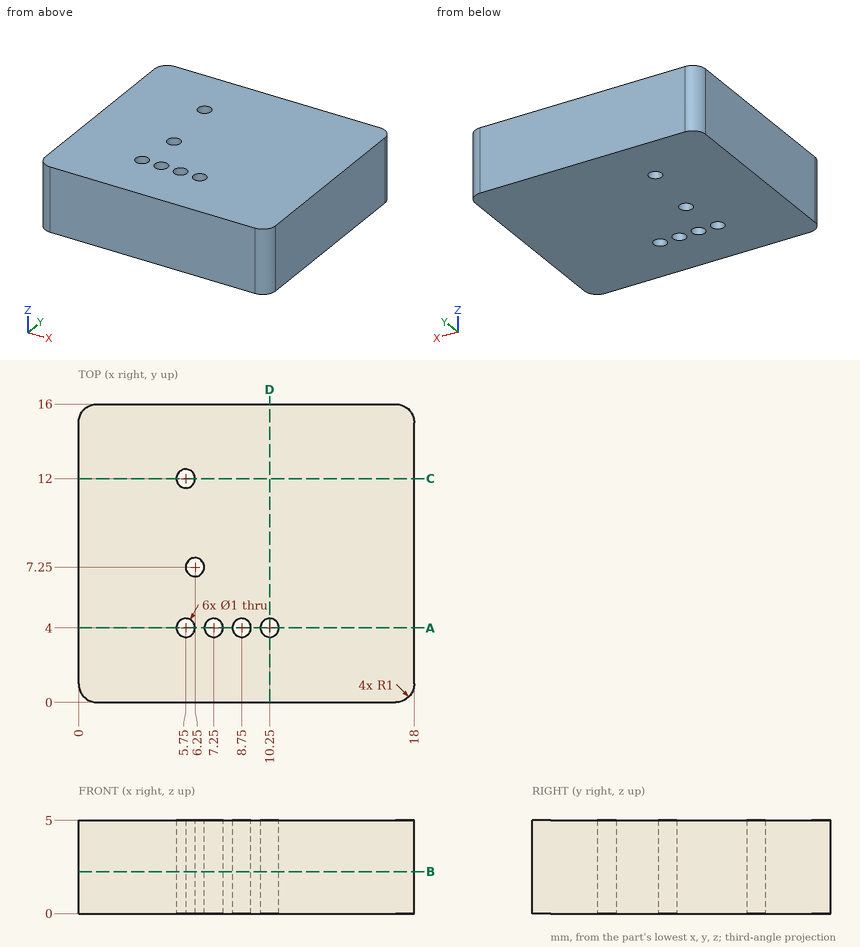
Job drawing, mm, ordinate dimensions from the low corner. One solid piece. Give positions to 0.01 mm unless a question says otherwise; leave off trailing zeros. Loops run counter-clockwise (first coordinate to the right, second up) from the corner with the lowest first, then second, coordinate; pieces in that order, holes last.
Item 1: Slice it at A-A, the plane y = 4. List the corners of the cut face in (x, z).
Answers follow:
outline: (0, 0) - (5.25, 0) - (5.25, 5) - (0, 5) - close; (6.25, 0) - (6.75, 0) - (6.75, 5) - (6.25, 5) - close; (7.75, 0) - (8.25, 0) - (8.25, 5) - (7.75, 5) - close; (9.25, 0) - (9.75, 0) - (9.75, 5) - (9.25, 5) - close; (10.75, 0) - (18, 0) - (18, 5) - (10.75, 5) - close
Item 2: Slice it at D-D, the plane x = 10.25. List the corners of the cut face in (y, z), and give its area (3 significant figures).
Answers follow:
outline: (0, 0) - (3.5, 0) - (3.5, 5) - (0, 5) - close; (4.5, 0) - (16, 0) - (16, 5) - (4.5, 5) - close
area: 75.0 mm2
Item 3: Slice it at C-C, the plane y = 12. List the corners of the cut face in (x, z), and give its area (3 significant figures).
Answers follow:
outline: (0, 0) - (5.25, 0) - (5.25, 5) - (0, 5) - close; (6.25, 0) - (18, 0) - (18, 5) - (6.25, 5) - close
area: 85.0 mm2
Item 4: Drill centre line: line 1 (X direction, y = 7.5, z = 4.2). Where is it in solid material? Low to high.
Answers follow:
line 1: x = 0 to 5.82, 6.68 to 18
Item 5: Slice it at B-B, the plane z = 2.25. List the corners of the cut face in (x, y).
Answers follow:
outline: (0, 1) arc R1 ccw to (1, 0) - (17, 0) arc R1 ccw to (18, 1) - (18, 15) arc R1 ccw to (17, 16) - (1, 16) arc R1 ccw to (0, 15) - close; hole circle Ø1 at (5.75, 4); hole circle Ø1 at (5.75, 12); hole circle Ø1 at (6.25, 7.25); hole circle Ø1 at (7.25, 4); hole circle Ø1 at (8.75, 4); hole circle Ø1 at (10.25, 4)
